```python
from build123d import *

# Parameters (mm, degrees)
F0_W     = 38
F0_H     = 20
F0_W_2   = 2.5
F0_H_2   = 8
F0_R     = 2.25
F1_DEPTH = 3.5
F2_W     = 5
F2_H     = 5.5
F3_DEPTH = 5.5
F4_R     = 2.49999


# Not quite as in the source:
# - a fillet or chamfer is up to 0.001 mm smaller than in the source, because OpenCascade refuses the exact size


with BuildPart() as f1:
    # F0 (on Top) → F1 (new body)
    with BuildSketch(Plane.XY):
        with Locations((11, -10)):
            Rectangle(F0_W, F0_H)
        with Locations((-3.3499999251, -10)):
            Rectangle(F0_W_2, F0_H_2, mode=Mode.SUBTRACT)
        with Locations((3, -10)):
            Circle(F0_R, mode=Mode.SUBTRACT)
        with Locations((10.75, -10)):
            Rectangle(F0_W_2, F0_H_2, mode=Mode.SUBTRACT)
        with Locations((18.25, -10)):
            Rectangle(F0_W_2, F0_H_2, mode=Mode.SUBTRACT)
        Polygon((24.5, -10), (24.5, -6), (27, -6), (27, -14), (24.5, -14), align=None, mode=Mode.SUBTRACT)
    extrude(amount=F1_DEPTH)

    # F2 (on face) → F3 (join)
    with BuildSketch(Plane.XY.offset(3.5)):
        with Locations((22, -10)):
            Rectangle(F2_W, F2_H)
        with Locations((14.5, -10)):
            Rectangle(F2_W, F2_H)
    extrude(amount=F3_DEPTH)

    # F4 (radius 2.5 in the source; OpenCascade refuses exactly that, so slightly less here)
    f4_edges = [f1.edges().sort_by_distance(p)[0] for p in [
        (12, -10, 9),
        (17, -10, 9),
        (19.5, -10, 9),
        (24.5, -10, 9),
    ]]
    fillet(f4_edges, radius=F4_R)


solid = f1.part
```
Check sheet for the modelled part. Datum: model origin and axes. Units: mm. A direction names the side the tool comes from. Round coordinates to 2 decimals unless told otherwise and drop trailing zeros. Order: outer loops, then holes, each group sorted by start corner. A loop starts at its lowest first (then second) coordinate and runs counter-clockwise, first axis right, second up.
1) Go/stop test with flat-tipped pins: pin 1 Ø5 at (y, z) = (-5.5, 7) entering from +X; pin 2 Ø1 at (x, z) = (18.5, 8) entering from +Y; pin 3 Ø1.5 at (x, z) = (21.5, 5.5) entering from -Y; pin 4 Ø6 at (x, y) = (1, -12) entering from +Z. Record where each tip stops, or that it passes through.
2) Section check D-D (z = 1.25). Record the boundary of the cut face in (x, y).
3) Section check A-A (z = 4). Record the boundary of the cut face in (x, y), and give its area (3 significant figures).
4) Scan lines: line 1 (Y direction, x = 3, z = 2.6); line 2 (X direction, y = -7.5, z = 5.25); line 3 (X direction, y = -10.5, z = 3.25). Record each from-to range of solid material in increasing order.
5) Tool access check on faces 1 (the flat face through (17, -10, 3)), 2 (the cylindrical face through (16.287, -9.962, 8.248)), 3 (the flat face through (22, -7.25, 6)), 4 (the flat face through (30, -10, 2)), 5 (the flat face through (7, -10, 0)). Record the directions out of +Z, -Z, +X, -X, +Y, -Y that give a thin tool (end or side, any length) a straight path to the whole face; none if there is none.
6) Mould release check, pull along X, two halves, no side actions. Record for faces 6 (the cylindrical face through (12.713, -9.962, 8.248)), 7 (the flat face through (26, -6, 2)), 8 (the flat face through (11, 0, 2)): +X half, -X half, draft (parallel to the pull), parting line (faces both ways), or undercut.
7) Section check B-B (y = -10). Give the number of separate pieces and of enclosed holes in the cut face, and give its area (3 significant figures).
8) Section check C-C (x = 10). Record the boundary of the cut face in (y, z).
Result:
1. pin 1: stops at x = 24.5
1. pin 2: passes through
1. pin 3: stops at y = -12.75
1. pin 4: stops at z = 3.5
2. outline: (-8, -20) - (30, -20) - (30, 0) - (-8, 0) - close; hole (-4.6, -14) - (-2.1, -14) - (-2.1, -6) - (-4.6, -6) - close; hole circle Ø4.5 at (3, -10); hole (9.5, -14) - (12, -14) - (12, -6) - (9.5, -6) - close; hole (17, -14) - (19.5, -14) - (19.5, -6) - (17, -6) - close; hole (24.5, -14) - (27, -14) - (27, -6) - (24.5, -6) - close
3. outline: (12, -12.75) - (17, -12.75) - (17, -7.25) - (12, -7.25) - close; (19.5, -12.75) - (24.5, -12.75) - (24.5, -7.25) - (19.5, -7.25) - close
3. area: 55.0 mm2
4. line 1: y = -20 to -12.25, -7.75 to 0
4. line 2: x = 12 to 17, 19.5 to 24.5
4. line 3: x = -8 to -4.6, -2.1 to 0.81, 5.19 to 9.5, 12 to 17, 19.5 to 24.5, 27 to 30
5. face 1: +Z, -Z
5. face 2: +Z, +Y, -Y
5. face 3: +Z, +X, -X, +Y
5. face 4: +Z, -Z, +X, +Y, -Y
5. face 5: -Z, +X, -X, +Y, -Y
6. face 6: -X half
6. face 7: undercut
6. face 8: draft
7. separate pieces: 6
7. enclosed holes: 0
7. area: 132 mm2
8. outline: (-20, 0) - (-14, 0) - (-14, 3.5) - (-20, 3.5) - close; (-6, 0) - (0, 0) - (0, 3.5) - (-6, 3.5) - close
